```python
from build123d import *

# Parameters (mm, degrees)
BOSS_EXTRUDE1_DEPTH   = 2
F_4_0MM_DOWEL_HOLE1_D = 4
CUT_EXTRUDE1_REACH    = 98.322
BOSS_EXTRUDE2_DEPTH   = 2


with BuildPart() as part:
    # Sketch2 → Boss-Extrude1 (new body)
    with BuildSketch(Plane.XY):
        Polygon((2, 9), (-54, 9), (-54, -5), (-74, -5), (-74, 2), (-93, 2), (-93, -20.44151844), (-79.32455532, -25), (-11.67544468, -25), (2, -20.44151844), align=None)
    extrude(amount=-BOSS_EXTRUDE1_DEPTH)

    # Ø4.0mm Dowel Hole1 (through all)
    with Locations(Plane.XY):
        with Locations((-40.5, 5), (-22.5, 5), (-4.5, 5)):
            Hole(F_4_0MM_DOWEL_HOLE1_D / 2)

    # Sketch1 → Cut-Extrude1 (cut, up to next)
    with BuildSketch(Plane.XY, mode=Mode.PRIVATE) as cut_extrude1_sk1:
        Polygon((0, 0), (0, -19), (-12, -23), (-79, -23), (-91, -19), (-91, 0), (-76, 0), (-76, -7), (-52, -7), (-52, 0), align=None)
    cut_extrude1_tool1 = extrude(cut_extrude1_sk1.sketch, amount=-CUT_EXTRUDE1_REACH, mode=Mode.PRIVATE) & part.part
    add(cut_extrude1_tool1.solids().sort_by_distance((-43.844166, -11.956047, 0))[0], mode=Mode.SUBTRACT)

    # Sketch5 → Boss-Extrude2 (add)
    with BuildSketch(Plane.XY):
        Polygon((-52, -7), (-52, -23), (-79, -23), (-91, -19), (-91, 0), (-76, 0), (-76, -7), align=None)
    extrude(amount=-BOSS_EXTRUDE2_DEPTH)


solid = part.part
```
Model file for the job. Use its own axes, mm. A direction names the side the tool comes from. Coordinates: 2 decimals unless noted, no trailing zeros. Order: outer loops, then holes, each group sorted by start corner. A loop starts at its lowest first (then second) coordinate and runs counter-clockwise, first axis right, second up. Notation, with made-up numbers: (-12.5, 8.25) -> (15.5, 8.25) arc R9 cw to (15.5, 22.25) -> close; hole circle Ø8 at (27.25, 39). An arc over 180 degrees is marked (long way). Answer as a JSON object with one key per item and string values. Group by question number.
1) Cut at B-B, the plane z = -1.35. Write the cut outline in (x, y).
2) Drill centre lines: L1, parallel to Y at x = -22.5, z = -0.8; L2, parallel to X at y = -1, z = -0.45; L3, parallel to Y at x = -17, z = -0.55. Where is each one in solid material? Low to high.
3) Cut at A-A, the plane y = -16. Write the cut outline in (x, z).
4) Which spindle directions (+Z, -Z, +X, -X, +Y, -Y) get a long thin tool onto all of the face, cutting with end or side? Do faces 1 (the face through (-54, 2, -1)), 2 (the face through (-32, -23, -1)), 3 (the face through (-93, -9, -1)). Say none if no direction does.
5) Cut at D-D, the plane y = -3. Write the cut outline in (x, z), then the cut area to 3 significant figures.
6) Pull direction Y, two halves, no side cores. Call faces 4 (the face through (-83, 2, -1)), 5 (the face through (-4.93, -22.75, -0.99)), 6 (the face through (-20.502, 5.088, -1.014)), 7 (the face through (-6, -21, -1)): +Y half, -Y half, draft (parallel to the pull), parting line (faces both ways), or undercut.
7) Flat gauge pins, fed straight in: pin 1 (0.6 mm diameter, centred on x = -66.5, z = -0.5, fed in from +Y); pin 2 (5 mm diameter, centred on x = -40.5, y = 5, fed in from +Z); pin 3 (2.5 mm diameter, centred on x = -22.5, y = 5, fed in from +Z). Where does each tip first touch, or does it go through?
8) Cut at C-C, the plane x = -40.5. Write the cut outline in (y, z).
Check values:
{
 "1": {"outline": "(-93, -20.44) -> (-79.32, -25) -> (-11.68, -25) -> (2, -20.44) -> (2, 9) -> (-54, 9) -> (-54, -5) -> (-74, -5) -> (-74, 2) -> (-93, 2) -> close; hole (-52, -23) -> (-12, -23) -> (0, -19) -> (0, 0) -> (-52, 0) -> close; hole circle Ø4 at (-40.5, 5); hole circle Ø4 at (-22.5, 5); hole circle Ø4 at (-4.5, 5)"},
 "2": {"L1": "y = -25 to -23, 0 to 3, 7 to 9", "L2": "x = -93 to -74, -54 to -52, 0 to 2", "L3": "y = -25 to -23, 0 to 9"},
 "3": {"outline": "(-93, -2) -> (-52, -2) -> (-52, 0) -> (-93, 0) -> close; (0, -2) -> (2, -2) -> (2, 0) -> (0, 0) -> close"},
 "4": {"face 1": "+Z, -Z, +Y", "face 2": "+Z, -Z", "face 3": "+Z, -Z, -X, +Y, -Y"},
 "5": {"outline": "(-93, -2) -> (-74, -2) -> (-74, 0) -> (-93, 0) -> close; (-54, -2) -> (-52, -2) -> (-52, 0) -> (-54, 0) -> close; (0, -2) -> (2, -2) -> (2, 0) -> (0, 0) -> close", "area": "46.0 mm²"},
 "6": {"face 4": "+Y half", "face 5": "-Y half", "face 6": "undercut", "face 7": "undercut"},
 "7": {"pin 1": "stops at y = -5", "pin 2": "stops at z = 0", "pin 3": "passes through"},
 "8": {"outline": "(-25, -2) -> (-23, -2) -> (-23, 0) -> (-25, 0) -> close; (0, -2) -> (3, -2) -> (3, 0) -> (0, 0) -> close; (7, -2) -> (9, -2) -> (9, 0) -> (7, 0) -> close"}
}
